For this review, use the dimensioned drawing (mm, ordinates from the lowest corner) and the shaded views. A direction names the side the tool comes from. Round coordinates to 2 decimals unless told otherwise and drop trailing zeros. Write each loop counter-clockwise with the first axis right and the second up, starting at its lowest first coordinate (ties: lowest second). Pieces come first, ordered by that corner, then holes.
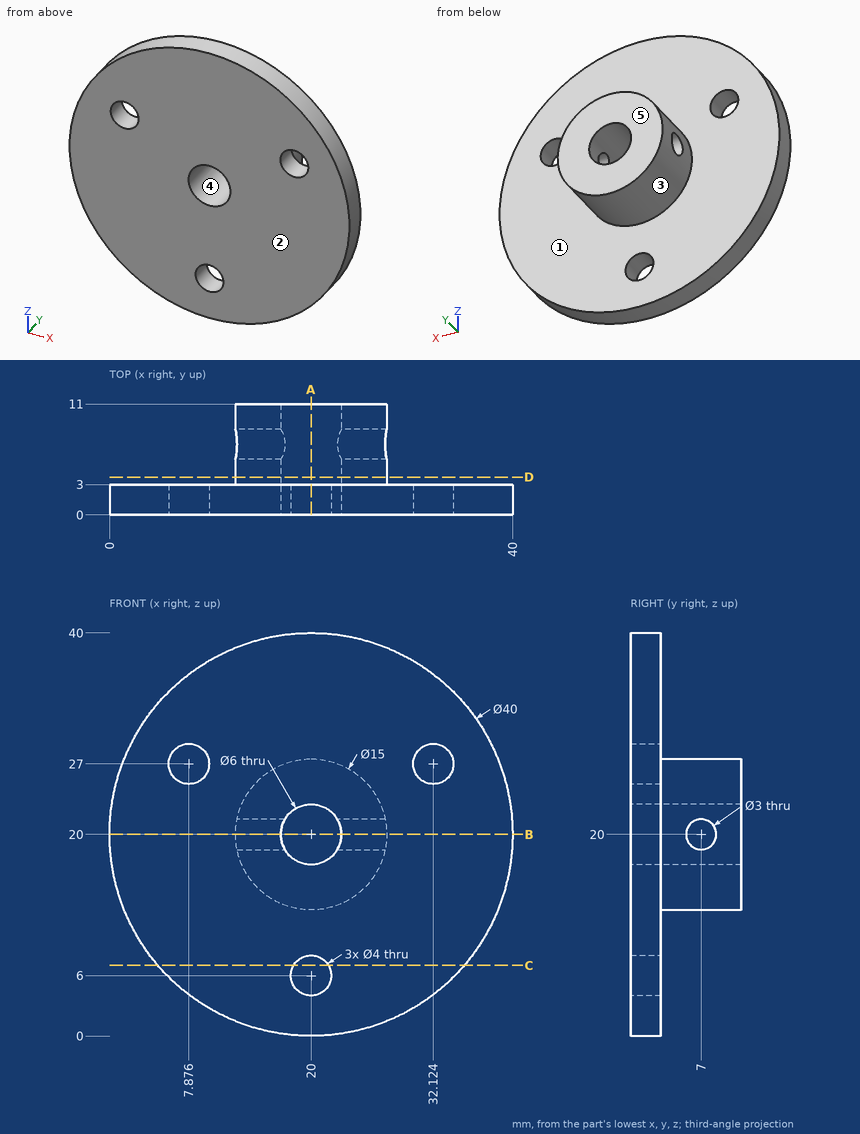
(1) We need section A-A, the plane x = 20. Give the boundary of the cut face in (y, z), and give its area (3 significant figures).
Geometry check:
outline: (0, 0) - (3, 0) - (3, 4) - (0, 4) - close; (0, 8) - (3, 8) - (3, 12.5) - (11, 12.5) - (11, 17) - (0, 17) - close; (0, 23) - (11, 23) - (11, 27.5) - (3, 27.5) - (3, 40) - (0, 40) - close
area: 162 mm2
(2) We need section C-C, the plane z = 7. Give the boundary of the cut face in (x, y), and give its area (3 significant figures).
Geometry check:
outline: (4.8, 0) - (18.27, 0) - (18.27, 3) - (4.8, 3) - close; (21.73, 0) - (35.2, 0) - (35.2, 3) - (21.73, 3) - close
area: 80.8 mm2
(3) For line 1 along X through (y, z) = (5.25, 20); line 2 along X through (y, z) = (1, 20); line 3 along X through (y, z) = (2, 26) (1 decimal), list the stretches that pass through material, from the lowest coordinate up.
Geometry check:
line 1: x = 12.5 to 17, 23 to 27.5
line 2: x = 0 to 17, 23 to 40
line 3: x = 0.9 to 6.1, 9.6 to 30.4, 33.9 to 39.1
(4) We need section B-B, the plane z = 20. Give the boundary of the cut face in (x, y), and give its area (3 significant figures).
Geometry check:
outline: (0, 0) - (17, 0) - (17, 5.5) - (12.5, 5.5) - (12.5, 3) - (0, 3) - close; (12.5, 8.5) - (17, 8.5) - (17, 11) - (12.5, 11) - close; (23, 0) - (40, 0) - (40, 3) - (27.5, 3) - (27.5, 5.5) - (23, 5.5) - close; (23, 8.5) - (27.5, 8.5) - (27.5, 11) - (23, 11) - close
area: 147 mm2
(5) For pin 1 Ø4.5 at (x, z) = (32.12, 27) entering from +Y; pin 2 Ø4 at (y, z) = (7, 20) entering from -X, all flat-tipped, find the tip position at first contact; note any pin that passes through.
Geometry check:
pin 1: stops at y = 3
pin 2: stops at x = 12.5
(6) We need section D-D, the plane y = 3.75. Give the boundary of the cut face in (x, z).
Geometry check:
outline: circle Ø15 at (20, 20); hole circle Ø6 at (20, 20)
(7) Mouldability with a two-part tool opening along Z and no side actions: class the marked faces 3, 4 and 5 as pulls with the +Z half, pulls with the -Z half, needs draft (parallel to the pull), parting line crosses it, or undercut.
Geometry check:
face 3: parting line crosses it
face 4: undercut
face 5: needs draft
(8) For the marked faces 1 and 2, list the 3-axis set-ups (+Z, -Z, +X, -X, +Y, -Y) from which the entire face can be reached by the end or side of a thin tool; tool diameter is ignored.
Geometry check:
face 1: +Y
face 2: +Z, -Z, +X, -X, -Y
